Here's how the part is built. I have some questions about the finished solid (model axes, mm). A direction names the side the tool comes from. Round coordinates to 2 decimals unless told otherwise and drop trailing zeros. Loops run counter-clockwise (first coordinate to the right, second up) from the corner with the lowest first, then second, coordinate; pieces in that order, holes last. Notation, with made-up numbers: M 51.5,3.25 L 86.5,3.25 A18 cw 86.5,30.25 Z; hole C 78,71 d3. An arc over 180 degrees is marked long. Write item = value, one per line. Start each with the question number.
from build123d import *

# Parameters (mm, degrees)
F0_W     = 60
F0_H     = 50
F0_W_2   = 55
F0_H_2   = 45
F1_DEPTH = 4
F3_DEPTH = 2.5
F5_DEPTH = 2.5


with BuildPart() as f1:
    # F0 (on Top) → F1 (new body)
    with BuildSketch(Plane.XY):
        Rectangle(F0_W, F0_H)
        Rectangle(F0_W_2, F0_H_2, mode=Mode.SUBTRACT)
    extrude(amount=F1_DEPTH)

    # F2 (on face) → F3 (join)
    with BuildSketch(Plane(origin=(-30, 0, 0), x_dir=(0, -1, 0), z_dir=(-1, 0, 0))):
        Polygon((-8, 12), (-8, 4), (8, 4), (8, 12), (0, 8), align=None)
    extrude(amount=-F3_DEPTH)

    # F4 (on face) → F5 (join)
    with BuildSketch(Plane.YZ.offset(30)):
        Polygon((-7.976269, 11.944397), (-7.976269, 4), (7.995203, 4), (7.995203, 11.999263), (0, 7.997541), align=None)
    extrude(amount=-F5_DEPTH)


solid = f1.part
Item 1: We'd pull the mould along X, two halves only. Please class faces 6 (the flat face through (-30, 0, 3)), 7 (the flat face through (0, 23, 4)), 8 (the flat face through (0, -22.5, 2)): released by +X, released by -X, zero draft, split by the parting line, or undercut.
Item 2: I want a section at A-A, the plane y = 17. List the corners of the cut face in (x, z) for me, then the cut area to 3 significant figures.
Item 3: For faces 1 (the flat face through (0, 22.5, 2)), 2 (the flat face through (-29, 4, 10)), 3 (the flat face through (-2, -24, 0)), 4 (the flat face through (-29, 8, 8)), 5 (the flat face through (-29, -8, 8)), which set-ups out of +Z, -Z, +X, -X, +Y, -Y let a thin tool reach every point of the face, with its end or its side?
Item 4: Please list where these lines run through material, in increasing order: line 1 (Y direction, x = -22.5, z = 1.5); line 2 (X direction, y = 2.5, z = 3.25). Write a range as [from, to].
Item 5: I want a section at C-C, the plane z = 10.5. List the corners of the cut face in (x, y) for me, then the cut area to 3 significant figures.
Item 6: Will these pins go through, and if not, where does the flat tip stop? pin 1 Ø0.8 at (x, z) = (-28, 8) entering from -Y; pin 2 Ø3 at (x, z) = (-29, 10) entering from +Y; pin 3 Ø13.5 at (x, y) = (-10, -18) entering from +Z.
Item 7: I want a section at B-B, the plane z = 6.25. List the corners of the cut face in (x, y) for me, then the cut area to 3 significant figures.
Worked out:
q1.face_6 = released by -X
q1.face_7 = zero draft
q1.face_8 = undercut
q2.outline = M -30,0 L -27.5,0 L -27.5,4 L -30,4 Z; M 27.5,0 L 30,0 L 30,4 L 27.5,4 Z
q2.area = 20.0 mm2
q3.face_1 = +Z, -Z
q3.face_2 = +Z, +X, -X
q3.face_3 = -Z, +X, -X, +Y, -Y
q3.face_4 = +Z, +X, -X, +Y
q3.face_5 = +Z, +X, -X, -Y
q4.line_1 = [-25, -22.5], [22.5, 25]
q4.line_2 = [-30, -27.5], [27.5, 30]
q5.outline = M -30,-8 L -27.5,-8 L -27.5,-5 L -30,-5 Z; M -30,5 L -27.5,5 L -27.5,8 L -30,8 Z; M 27.5,-7.98 L 30,-7.98 L 30,-5.06 L 27.5,-5.06 Z; M 27.5,5 L 30,5 L 30,8 L 27.5,8 Z
q5.area = 29.8 mm2
q6.pin_1 = -8
q6.pin_2 = 8
q6.pin_3 = 4
q7.outline = M -30,-8 L -27.5,-8 L -27.5,8 L -30,8 Z; M 27.5,-7.98 L 30,-7.98 L 30,8 L 27.5,8 Z
q7.area = 79.9 mm2
